Build history of the part. All positions in model axes, mm. Give positions to 0.01 mm unless a question says otherwise; leave off trailing zeros. Answer in a Markdown table with one row per item. Add a question column.
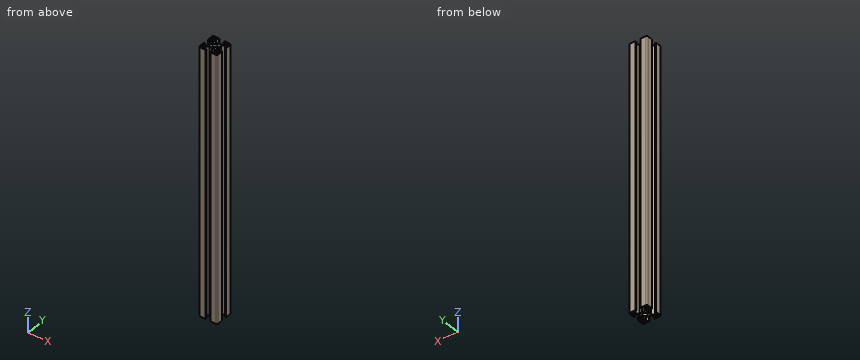
Autodesk Inventor part; units mm, degrees
ref_plane "C1_XY" through (0, 0, 0) normal (0, 0, 1) x (1, 0, 0)
ref_plane "C1_YZ" through (0, 0, 0) normal (1, 0, 0) x (0, 1, 0)
ref_plane "C1_ZX" through (0, 0, 0) normal (0, 1, 0) x (0, 0, 1)
sketch "Sketch_1" plane through (0, 0, 0) normal (0, 0, 1) x (1, 0, 0)
  line L0 (-15, -4) -> (-15, -13)
  arc A0 (-15, -13) -> (-13, -15) centre (-13, -13) ccw
  line L1 (-13, -15) -> (-4, -15)
  line L2 (-4, -15) -> (-4, -13)
  line L3 (-4, -13) -> (-8.25, -13)
  line L4 (-8.25, -13) -> (-8.25, -9.6642)
  line L5 (-8.25, -9.6642) -> (-4.5858, -6)
  line L6 (-4.5858, -6) -> (-0.5196, -6)
  line L7 (-0.5196, -6) -> (0, -5.7)
  line L8 (0, -5.7) -> (0.5196, -6)
  line L9 (0.5196, -6) -> (4.5858, -6)
  line L10 (4.5858, -6) -> (8.25, -9.6642)
  line L11 (8.25, -9.6642) -> (8.25, -13)
  line L12 (8.25, -13) -> (4, -13)
  line L13 (4, -13) -> (4, -15)
  line L14 (4, -15) -> (13, -15)
  arc A1 (13, -15) -> (15, -13) centre (13, -13) ccw
  line L15 (15, -13) -> (15, -4)
  line L16 (15, -4) -> (13, -4)
  line L17 (13, -4) -> (13, -8.25)
  line L18 (13, -8.25) -> (9.6642, -8.25)
  line L19 (9.6642, -8.25) -> (6, -4.5858)
  line L20 (6, -4.5858) -> (6, -0.5196)
  line L21 (6, -0.5196) -> (5.7, 0)
  line L22 (5.7, 0) -> (6, 0.5196)
  line L23 (6, 0.5196) -> (6, 4.5858)
  line L24 (6, 4.5858) -> (9.6642, 8.25)
  line L25 (9.6642, 8.25) -> (13, 8.25)
  line L26 (13, 8.25) -> (13, 4)
  line L27 (13, 4) -> (15, 4)
  line L28 (15, 4) -> (15, 13)
  arc A2 (15, 13) -> (13, 15) centre (13, 13) ccw
  line L29 (13, 15) -> (4, 15)
  line L30 (4, 15) -> (4, 13)
  line L31 (4, 13) -> (8.25, 13)
  line L32 (8.25, 13) -> (8.25, 9.6642)
  line L33 (8.25, 9.6642) -> (4.5858, 6)
  line L34 (4.5858, 6) -> (0.5196, 6)
  line L35 (0.5196, 6) -> (0, 5.7)
  line L36 (0, 5.7) -> (-0.5196, 6)
  line L37 (-0.5196, 6) -> (-4.5858, 6)
  line L38 (-4.5858, 6) -> (-8.25, 9.6642)
  line L39 (-8.25, 9.6642) -> (-8.25, 13)
  line L40 (-8.25, 13) -> (-4, 13)
  line L41 (-4, 13) -> (-4, 15)
  line L42 (-4, 15) -> (-13, 15)
  arc A3 (-13, 15) -> (-15, 13) centre (-13, 13) ccw
  line L43 (-15, 13) -> (-15, 4)
  line L44 (-15, 4) -> (-13, 4)
  line L45 (-13, 4) -> (-13, 8.25)
  line L46 (-13, 8.25) -> (-9.6642, 8.25)
  line L47 (-9.6642, 8.25) -> (-6, 4.5858)
  line L48 (-6, 4.5858) -> (-6, 0.5196)
  line L49 (-6, 0.5196) -> (-5.7, 0)
  line L50 (-5.7, 0) -> (-6, -0.5196)
  line L51 (-6, -0.5196) -> (-6, -4.5858)
  line L52 (-6, -4.5858) -> (-9.6642, -8.25)
  line L53 (-9.6642, -8.25) -> (-13, -8.25)
  line L54 (-13, -8.25) -> (-13, -4)
  line L55 (-13, -4) -> (-15, -4)
extrude "Extrusion1" add sketch "Sketch_1" against normal blind 440
sketch "Sketch2" plane through (0, 0, -440) normal (0, 0, -1) x (-1, 0, 0)
  point P0 (0, 0)
hole "Hole1" at (0, 0, -440) direction (0, 0, 1) diameter 6.8 depth 440
sketch "Sketch3" plane through (0, 0, -440) normal (0, 0, -1) x (-1, 0, 0)
  point P0 (-11.6, 11.6)
hole "Hole2" at (11.6, 11.6, -440) direction (0, 0, 1) diameter 4.2 depth 440
pattern_linear "Rectangular Pattern1" count 2 spacing 23.2 along (-1, 0, 0) count 2 spacing 23.2 along (0, -1, 0) of "Hole2"
ref_plane "C1_XY" through (0, 0, 0) normal (0, 0, 1) x (1, 0, 0)
ref_plane "C1_YZ" through (0, 0, 0) normal (1, 0, 0) x (0, 1, 0)
ref_plane "C1_ZX" through (0, 0, 0) normal (0, 1, 0) x (0, 0, 1)
ref_plane "to_frame_cap1_XY" through (0, 0, 0) normal (0, 0, 1) x (1, 0, 0)
ref_plane "to_frame_cap1_YZ" through (0, 0, 0) normal (1, 0, 0) x (0, 1, 0)
ref_plane "to_frame_cap1_ZX" through (0, 0, 0) normal (0, 1, 0) x (0, 0, 1)
ref_plane "to_frame_cap2_XY" through (0, 0, -440) normal (0, 0, -1) x (1, 0, 0)
ref_plane "to_frame_cap2_YZ" through (0, 0, -440) normal (1, 0, 0) x (0, -1, 0)
ref_plane "to_frame_cap2_ZX" through (0, 0, -440) normal (0, -1, 0) x (0, 0, -1)
properties part number "HFS6-3030-440"
(1) Pin check, flat tips, straight feed: pin 1 (2 mm diameter, centred on y = -14.5, z = -290, fed in from +X); pin 2 (0.6 mm diameter, centred on y = -14, z = -190.5, fed in from -X); pin 3 (2 mm diameter, centred on x = -2.5, z = -260.5, fed in from +Y). Stop position of each tip, or through.
(2) Slice it at A-A, the plane z = -162. State how many separate pieces and enclosed holes the cut face has, then the cut area to 3 significant figures.
(3) Wall check: line 1 (Y direction, x = 11.6, z = -292); line 2 (Y direction, x = 0, z = -239). Give the ranges that are in metal, low to high.
Solution:
| question | item | result |
|---|---|---|
| 1 | pin 1 | x = 14.94 |
| 1 | pin 2 | x = -14.87 |
| 1 | pin 3 | y = 6 |
| 2 | separate pieces | 1 |
| 2 | enclosed holes | 5 |
| 2 | area | 332 mm^2 |
| 3 | line 1 | -15 to -13.7, -9.5 to -8.25, 8.25 to 9.5, 13.7 to 15 |
| 3 | line 2 | -5.7 to -3.4, 3.4 to 5.7 |
